Read the model definition and answer for the solid it produces. Units are mm, in the model's axes. A direction names the side the tool comes from. Coordinates: 2 decimals unless noted, no trailing zeros. Return JSON: item names as keys, results as strings.
from build123d import *

# Parameters (mm, degrees)
ESQUISSE1_W             = 46
ESQUISSE1_H             = 25.6
ESQUISSE1_R             = 1.7
ESQUISSE1_R_2           = 2.6
BOSS_EXTRU_1_DEPTH      = 5
ENL_V_MAT_EXTRU_2_DEPTH = 3
ENL_V_MAT_EXTRU_2_TAPER = 5
CONG_1_R                = 4


with BuildPart() as part:
    # Esquisse1 → Boss.-Extru.1 (new body)
    with BuildSketch(Plane.XY):
        with Locations((15.830047476, 0)):
            Rectangle(ESQUISSE1_W, ESQUISSE1_H)
        with Locations((0.830047476, 0)):
            Circle(ESQUISSE1_R, mode=Mode.SUBTRACT)
        with Locations((9.315328851, 8.485281374)):
            Circle(ESQUISSE1_R_2, mode=Mode.SUBTRACT)
        with Locations((9.315328851, -8.485281374)):
            Circle(ESQUISSE1_R_2, mode=Mode.SUBTRACT)
        with Locations((30.830047476, 0)):
            Circle(ESQUISSE1_R, mode=Mode.SUBTRACT)
    extrude(amount=BOSS_EXTRU_1_DEPTH)

    # Esquisse3 → Enlèv. mat.-Extru.2 (cut)
    with BuildSketch(Plane.XY.offset(5)):
        Polygon((4.063208984, 0), (2.44662823, 2.8), (-0.786533277, 2.8), (-2.403114031, 0), (-0.786533277, -2.8), (2.44662823, -2.8), align=None)
        Polygon((34.063208984, 0), (32.44662823, 2.8), (29.213466723, 2.8), (27.596885969, 0), (29.213466723, -2.8), (32.44662823, -2.8), align=None)
    extrude(amount=-ENL_V_MAT_EXTRU_2_DEPTH, taper=ENL_V_MAT_EXTRU_2_TAPER, mode=Mode.SUBTRACT)

    # Congé1
    cong_1_edges = [part.edges().sort_by_distance(p)[0] for p in [
        (38.830047476, -12.8, 2.5),
        (-7.169952524, -12.8, 2.5),
        (-7.169952524, 12.8, 2.5),
        (38.830047476, 12.8, 2.5),
    ]]
    fillet(cong_1_edges, radius=CONG_1_R)


solid = part.part
1. A tool of negligible diameter and unlimited length cuts with its end or side. For faces 1 (the face through (0.46, -1.66, 0.99)), 2 (the face through (31, 2, 2)), from which of +Z, -Z, +X, -X, +Y, -Y can it reach the whole face along a straight path? Write none if from no direction.
Taken from the geometry:
{"face 1": "+Z, -Z", "face 2": "+Z"}
2. Consider L1, parallel to X at y = 0, z = 0.6; L2, parallel to X at y = 2, z = 2.3; L3, parallel to X at y = 8.5, z = 3.15. Determine where each line is inside the solid, lowest interval first.
Taken from the geometry:
{"L1": "x = -7.17 to -0.87, 2.53 to 29.13, 32.53 to 38.83", "L2": "x = -7.17 to -0.98, 2.64 to 29.02, 32.64 to 38.83", "L3": "x = -7.17 to 6.72, 11.92 to 38.83"}
3. A flat-ended cylindrical pin translates along its axis: pin 1 Ø7 at (x, y) = (9.32, -8.49) entering from -Z. Find the tip coordinate at first contact, or state that the pin passes through.
Taken from the geometry:
{"pin 1": "stops at z = 0"}
4. The part is cut by section A-A (z = 4.2). Count the separate pieces of the cut face and the enclosed holes in it, then the cut area to 3 significant figures.
Taken from the geometry:
{"separate pieces": "1", "enclosed holes": "4", "area": "1,070 mm2"}
5. For a pull along Y with two mould halves and no side action, classify faces 3 (the face through (37.627, -11.659, 2.535)), 4 (the face through (1, -2, 2)), 5 (the face through (16, 0, 0)) as +Y half, -Y half, draft (parallel to the pull), parting line (faces both ways), or undercut.
Taken from the geometry:
{"face 3": "-Y half", "face 4": "undercut", "face 5": "draft"}
